Can you work these out from the model? Positions are in its coordinate system, mm. Face numbers are marked on the shaded views. A direction names the side the tool comes from. Give positions to 0.01 mm unless a question says otherwise; leave off trailing zeros. Loops run counter-clockwise (first coordinate to the right, second up) from the corner with the lowest first, then second, coordinate; pieces in that order, holes last. Notation, with made-up numbers: (-10, -35.5) - (7, -35.5) arc R23 cw to (7, -25.5) - close; hole circle Ø2 at (-9, 0). An arc over 180 degrees is marked (long way). Answer in a Markdown table with one row per item.
from build123d import *

# Parameters (mm, degrees)
SKETCH1_R           = 7.5
BOSS_EXTRUDE1_DEPTH = 5
SKETCH2_R           = 11
SKETCH2_R_2         = 7.5
BOSS_EXTRUDE2_DEPTH = 1


with BuildPart() as part:
    # Sketch1 → Boss-Extrude1 (new body, symmetric)
    with BuildSketch(Plane(origin=(0, 0, 0), x_dir=(1, 0, 0), z_dir=(0, 1, 0))):
        Circle(SKETCH1_R)
        Polygon((-2.893968224, -5.0125), (2.893968224, -5.0125), (5.787936449, 0), (2.893968224, 5.0125), (-2.893968224, 5.0125), (-5.787936449, 0), align=None, mode=Mode.SUBTRACT)
    extrude(amount=BOSS_EXTRUDE1_DEPTH, both=True)

    # Sketch2 → Boss-Extrude2 (add)
    with BuildSketch(Plane.XZ.offset(5)):
        Circle(SKETCH2_R)
        Circle(SKETCH2_R_2, mode=Mode.SUBTRACT)
    extrude(amount=-BOSS_EXTRUDE2_DEPTH)


solid = part.part
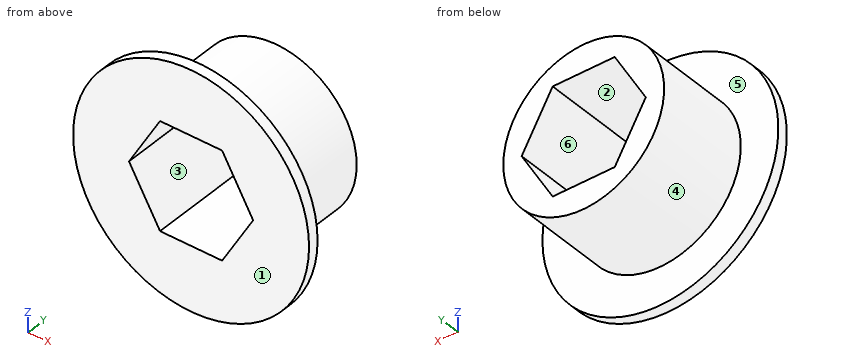
Q1. For pin 1 (1.7 mm diameter, centred on x = -1, y = -1.5, fed in from +Z); pin 2 (4 mm diameter, centred on y = -4, z = -2.5, fed in from +X); pin 3 (6 mm diameter, centred on x = -5.5, y = 3, fed in from +Z); pin 4 (6.5 mm diameter, centred on x = 3.5, z = 0.5, fed in from +Y), each with a flat end and sliding along its axis, tell me the tip position at first contact or that it passes through.
Checked values:
| item | result |
|---|---|
| pin 1 | stops at z = 7.5 |
| pin 2 | stops at x = 10.99 |
| pin 3 | stops at z = 7.07 |
| pin 4 | stops at y = 5 |
Q2. If we mould it in two halves opening along X, with no side actions, what happens to the marked faces 3, 4, 5 and 6? For each: released by +X, released by -X, zero draft, split by the parting line, or undercut.
Checked values:
| item | result |
|---|---|
| face 3 | undercut |
| face 4 | split by the parting line |
| face 5 | zero draft |
| face 6 | undercut |
Q3. Imagine slicing it at B-B, the plane x = 0. Write out the boundary of the cut face in (y, z).
Checked values:
| item | result |
|---|---|
| outline | (-5, -11) - (-4, -11) - (-4, -7.5) - (5, -7.5) - (5, -5.01) - (-5, -5.01) - close; (-5, 5.01) - (5, 5.01) - (5, 7.5) - (-4, 7.5) - (-4, 11) - (-5, 11) - close |
Q4. Imagine slicing it at A-A, the plane y = 1.75. Write out the boundary of the cut face in (x, z), and give its area (3 significant figures).
Checked values:
| item | result |
|---|---|
| outline | circle Ø15 at (0, 0); hole (-5.79, 0) - (-2.89, -5.01) - (2.89, -5.01) - (5.79, 0) - (2.89, 5.01) - (-2.89, 5.01) - close |
| area | 89.7 mm² |
Q5. Imagine slicing it at D-D, the plane x = -6.75. Write out the boundary of the cut face in (y, z).
Checked values:
| item | result |
|---|---|
| outline | (-5, -8.69) - (-4, -8.69) - (-4, -3.27) - (5, -3.27) - (5, 3.27) - (-4, 3.27) - (-4, 8.69) - (-5, 8.69) - close |
Q6. On a 3-axis mill with a long thin cutter (end or side, diameter ignored), from which of +Z, -Z, +X, -X, +Y, -Y can I reach the whole of each face in a straight line? I mean the marked faces 1 and 2. Say none if no direction works.
Checked values:
| item | result |
|---|---|
| face 1 | +Z, -Z, +X, -X, -Y |
| face 2 | +Y, -Y |
Q7. Imagine slicing it at C-C, the plane z = -1. Write out the boundary of the cut face in (x, y).
Checked values:
| item | result |
|---|---|
| outline | (-10.95, -5) - (-5.21, -5) - (-5.21, 5) - (-7.43, 5) - (-7.43, -4) - (-10.95, -4) - close; (5.21, -5) - (10.95, -5) - (10.95, -4) - (7.43, -4) - (7.43, 5) - (5.21, 5) - close |
Q8. If I drill on line 1 (Y direction, x = 8, z = -6); line 2 (Z direction, x = -3.75, y = -1); line 3 (Z direction, x = 3, y = -1), over which ranges is the centre line in solid material (lowest first)? Write a range as [from, to].
Checked values:
| item | result |
|---|---|
| line 1 | y = [-5, -4] |
| line 2 | z = [-6.5, -3.53], [3.53, 6.5] |
| line 3 | z = [-6.87, -4.83], [4.83, 6.87] |
